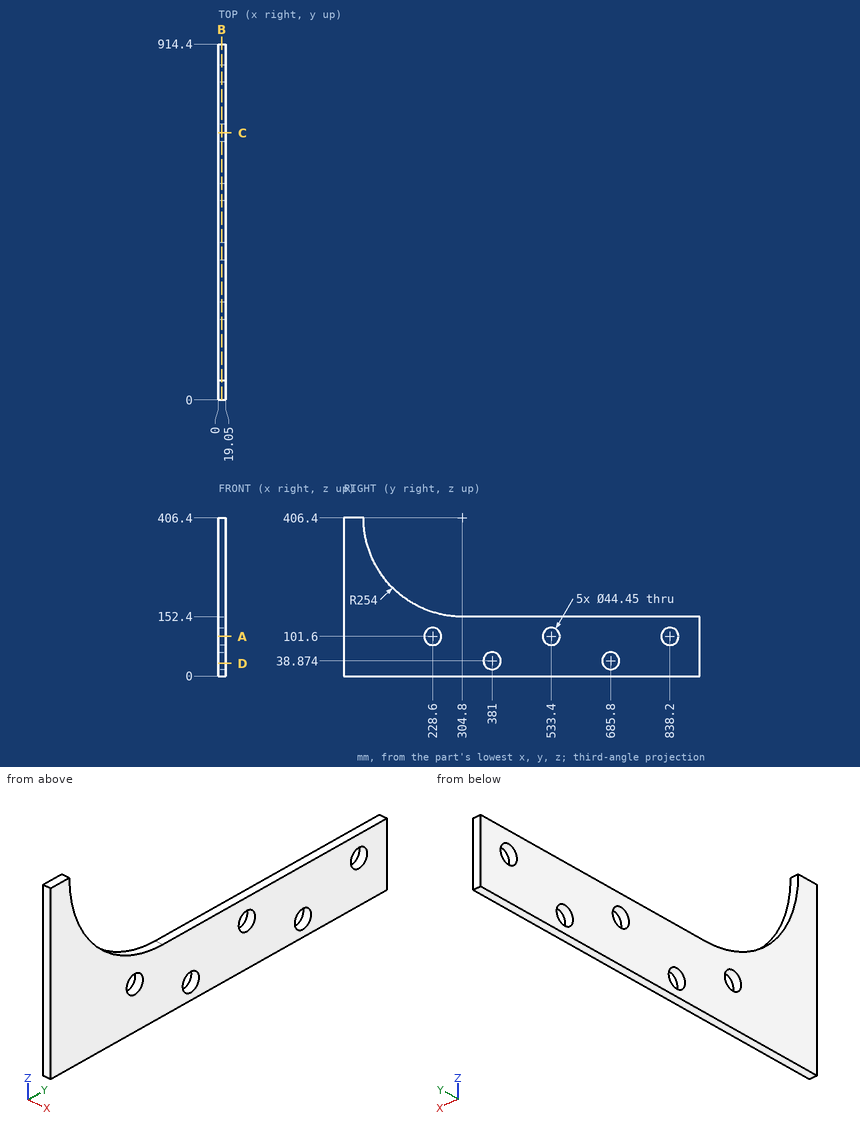
Can you work these out from the drawing? Everything is in mm from the part's minimum corner. Give positions to 0.01 mm unless a question says otherwise; leave off trailing zeros. Loops run counter-clockwise (first coordinate to the right, second up) from the corner with the lowest first, then second, coordinate; pieces in that order, holes last. Notation, with made-up numbers: M 80.5,8 L 123.5,8 A35 cw 123.5,45 Z; hole C 68,66.25 d11. An arc over 180 degrees is marked long. Put each result on its own line as item: value. Start each with the question number.
(1) I want a section at C-C on y = 685.8. Please give me the cut outline in (x, z), then the cut area to 3 significant figures.
(2) I need wall thicknesses on line 1 along Y through (x, z) = (11.5, 101.6) (3 decimals); line 2 along Z through (x, y) = (11, 685.8); line 3 along Y through (x, z) = (4, 84). Which ranges of each line are inside material? Lowest first, please. Write a range as [from, to].
(3) Will this pin go through, and if not, where does the flat tip stop? pin 1 Ø1 at (x, y) = (9, 812) entering from +Z.
(4) I want a section at D-D on z = 32.5. Please give me the cut outline in (x, y).
(5) I want a section at B-B on x = 8.25. State how many separate pieces and enclosed holes the cut face has, then the cut area to 3 significant figures.
(6) I want a section at A-A on z = 101.6. Please give me the cut outline in (x, y) (3 decimals).
Answer block:
1. outline: M 0,0 L 19.05,0 L 19.05,16.65 L 0,16.65 Z; M 0,61.1 L 19.05,61.1 L 19.05,152.4 L 0,152.4 Z
1. area: 2,060 mm^2
2. line 1: [0, 206.375], [250.825, 511.175], [555.625, 815.975], [860.425, 914.4]
2. line 2: [0, 16.65], [61.1, 152.4]
2. line 3: [0, 215.03], [242.17, 519.83], [546.97, 824.63], [851.77, 914.4]
3. pin 1: z = 152.4
4. outline: M 0,0 L 19.05,0 L 19.05,359.71 L 0,359.71 Z; M 0,402.29 L 19.05,402.29 L 19.05,664.51 L 0,664.51 Z; M 0,707.09 L 19.05,707.09 L 19.05,914.4 L 0,914.4 Z
5. separate pieces: 1
5. enclosed holes: 5
5. area: 158,000 mm^2
6. outline: M 0,0 L 19.05,0 L 19.05,206.375 L 0,206.375 Z; M 0,250.825 L 19.05,250.825 L 19.05,511.175 L 0,511.175 Z; M 0,555.625 L 19.05,555.625 L 19.05,815.975 L 0,815.975 Z; M 0,860.425 L 19.05,860.425 L 19.05,914.4 L 0,914.4 Z
